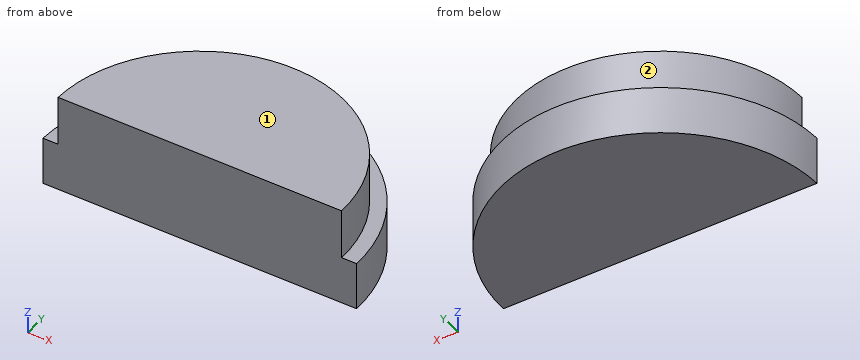
Solid Edge part; units mm, degrees
sketch "Sketch1" plane through (0, 0, 0) normal (0, 0, 1) x (1, 0, 0)
  arc A0 (-52, -26) -> (52, -26) centre (0, -26.2795) cw
  line L0 (-52, -26) -> (52, -26)
extrude "Protrusion1" add sketch "Sketch1" against normal blind 32
sketch "Sketch2" plane through (0, -0.1394, 0) normal (0, 0, 1) x (1, 0, 0)
  line L0 (-55.74, -28.2911) -> (55.74, -28.2911)
  line L1 (55.74, -28.2911) -> (55.74, 28.5699)
  line L2 (55.74, 28.5699) -> (-55.74, 28.5699)
  line L3 (-55.74, 28.5699) -> (-55.74, -28.2911)
extrude "Recorte_Extrudado_2" cut sketch "Sketch2" against normal blind 16.3
sketch "Sketch3" plane through (0, -0.1394, -16.3) normal (0, 0, 1) x (1, 0, 0)
  line L0 (-47, -25.8606) -> (47, -25.8606)
  arc A0 (-47, -25.8606) -> (47, -25.8606) centre (0, -25.8606) cw
extrude "Protrusão_Extrudada_5" add sketch "Sketch3" along normal blind 16.3
Geometry: final body of the model. Coordinates: model frame, mm. Face numbers are marked on the shaded views. A direction names the side the tool comes from. Coordinates: 2 decimals unless noted, no trailing zeros. Order: outer loops, then holes, each group sorted by start corner. A loop starts at its lowest first (then second) coordinate and runs counter-clockwise, first axis right, second up. Notation, with made-up numbers: (50.5, 7.25) - (95.5, 7.25) arc R18 cw to (95.5, 13.25) - close; hole circle Ø2 at (84.25, 23). An arc over 180 degrees is marked (long way). Return JSON: item names as keys, results as strings. Group by question number.
1. Cut plane C-C (z = -8.5). Output: boundary loops of the cut face in (x, y), plus the area to 3 significant figures.
2. Cut plane A-A (y = -4.5). Output: boundary loops of the cut face in (x, z).
3. Cut plane B-B (x = 0). Output: boundary loops of the cut face in (y, z).
4. Cut plane D-D (y = -14). Output: boundary loops of the cut face in (x, z).
5. Material intervals for line 1 along Z through (x, y) = (-33, 13.5); line 2 along X through (y, z) = (-13, -24); line 3 along Y through (x, z) = (-2, -29.5), sorted ascending. Write a range as [from, to].
6. Set-up query: the marked faces 1 and 2. Return all of +Z, -Z, +X, -X, +Y, -Y with unobstructed straight access to the full face (end or side cutting, diameter ignored); none if empty.
7. Pin query (flat end, axial travel): pin 1 (8 mm diameter, centred on y = -14, z = -3.5, fed in from +X); pin 2 (5 mm diameter, centred on y = -10, z = -20, fed in from +X); pin 3 (3 mm diameter, centred on x = 31, y = 16.5, fed in from -Z); pin 4 (4 mm diameter, centred on y = -3, z = -18, fed in from +X). Return the tip coordinate at first contact, or that it passes through.
Resolved:
{
 "1": {"outline": "(-47, -26) - (47, -26) arc R47 ccw to start", "area": "3,470 mm²"},
 "2": {"outline": "(-47.22, -32) - (47.22, -32) - (47.22, -16.3) - (41.79, -16.3) - (41.79, 0) - (-41.79, 0) - (-41.79, -16.3) - (-47.22, -16.3) - close"},
 "3": {"outline": "(-26, -32) - (25.72, -32) - (25.72, -16.3) - (21, -16.3) - (21, 0) - (-26, 0) - close"},
 "4": {"outline": "(-50.53, -32) - (50.53, -32) - (50.53, -16.3) - (45.44, -16.3) - (45.44, 0) - (-45.44, 0) - (-45.44, -16.3) - (-50.53, -16.3) - close"},
 "5": {"line 1": "z = [-32, -16.3]", "line 2": "x = [-50.28, 50.28]", "line 3": "y = [-26, 25.68]"},
 "6": {"face 1": "+Z, +X, -X, +Y, -Y", "face 2": "+Z, +Y"},
 "7": {"pin 1": "stops at x = 46.31", "pin 2": "stops at x = 50.14", "pin 3": "stops at z = -32", "pin 4": "stops at x = 47.45"}
}
